Source: CAD feature listing. Evaluate the final solid. Frame: model axes, mm. Face numbers are marked on the shaded views. A direction names the side the tool comes from. Round coordinates to 2 decimals unless told otherwise and drop trailing zeros. Loops run counter-clockwise (first coordinate to the right, second up) from the corner with the lowest first, then second, coordinate; pieces in that order, holes last.
Item 1: Section query A-A on z = 13.75. Return loops of the section in (x, y).
Item 2: Section query C-C on y = 9.5. Return loops of the section in (x, z).
Item 3: Section query D-D on x = -9. Return loops of the section in (y, z).
Item 4: First-contact query: P1, Ø5, axis at x = 2, y = 0.5, coming from the +Z side; P2, Ø4, axis at x = 36, y = 3, coming from the +Z side; P3, Ø8, axis at x = -15.5, z = 3, coming from the -Y side; P4, Ø1.5, axis at y = 7, z = 14, coming from the -X side. Flat tips, straight axial feed; report the tip coordinate or a pass-through.
Item 5: Ray query, L1, parallel to Y at x = -43.5, z = 2.1; L2, parallel to Y at x = -3, z = 13; L3, parallel to X at y = 1, z = 6.75. Return the intervals inside material, ascending.
Item 6: Section query B-B on x = -43.5. Return loops of the section in (y, z), then the cut area to 3 significant figures.
Item 7: Access query for the marked faces 1, 2 and 3. Directions: +Z, -Z, +X, -X, +Y, -Y. A direction counts if a zero-diameter tool reaches every point of the face in a straight line with its end or side. Return the directions, or none.
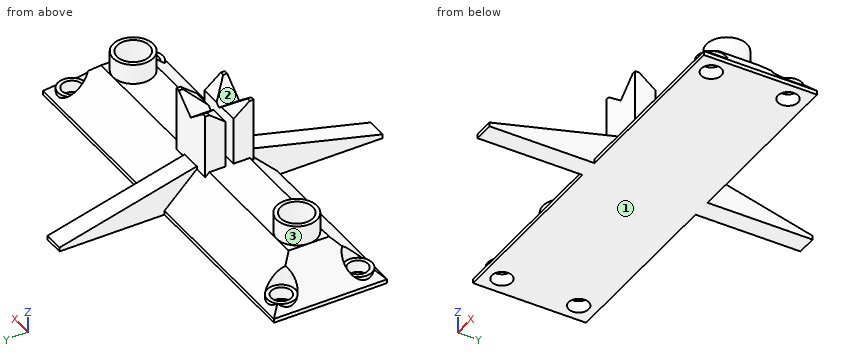
```python
from build123d import *

# Parameters (mm, degrees)
F0_R         = 3.5
F0_R_2       = 5
F0_W         = 5
F0_H         = 26
F0_W_2       = 2.5
F0_H_2       = 6
F0_W_3       = 3.5
F1_DEPTH     = 10
F0_R_3       = 4
F2_DEPTH     = 15
F3_DEPTH     = 1
F4_T4_DEPTH  = 74.2902937834
F4_S5_R      = 5
F4_T6_DEPTH  = 39
F4_T10_DEPTH = 74.2902937834
F4_S11_R     = 5
F4_T12_DEPTH = 39
F4_T16_DEPTH = 91.7902937834
F4_T21_DEPTH = 68.6451468917
F4_S22_R     = 5
F4_T23_DEPTH = 36
F4_T27_DEPTH = 68.6451468917
F4_S28_R     = 5
F4_T29_DEPTH = 36
F4_T33_DEPTH = 91.7902937834
F4_T38_DEPTH = 91.7902937834
F4_T43_DEPTH = 68.6451468917
F4_S44_R     = 5
F4_T45_DEPTH = 36
F4_T49_DEPTH = 68.6451468917
F4_S50_R     = 5
F4_T51_DEPTH = 36
F4_T55_DEPTH = 91.7902937834
F5_SIZE2     = 9
F5_SIZE      = 35
F0_R_4       = 2.5
F6_DEPTH     = 3
F7_DEPTH     = 25
F8_W         = 2
F8_H         = 7
F10_DEPTH    = 25
F11_DEPTH    = 25


# Not quite as in the source:
# - a fillet or chamfer that OpenCascade refuses, or shapes differently, is made with other operations: its cross-section is extruded or revolved along the edge and cut away or added


with BuildPart() as f1:
    # F0 (on Top) → F1 (new body)
    with BuildSketch(Plane.XY):
        Polygon((-2.5, 14), (-48, 14), (-48, -14), (-2.5, -14), (-2.5, -6), (-6, -6), (-6, 0), (-6, 6), (-2.5, 6), align=None)
        with Locations((-43.5, -9.5)):
            Circle(F0_R, mode=Mode.SUBTRACT)
        with Locations((-43.5, 9.5)):
            Circle(F0_R, mode=Mode.SUBTRACT)
        with Locations((-34, 0)):
            Circle(F0_R_2, mode=Mode.SUBTRACT)
        Polygon((48, 14), (2.5, 14), (2.5, 6), (6, 6), (6, 0), (6, -6), (2.5, -6), (2.5, -14), (48, -14), align=None)
        with Locations((43.5, -9.5)):
            Circle(F0_R, mode=Mode.SUBTRACT)
        with Locations((34, 0)):
            Circle(F0_R_2, mode=Mode.SUBTRACT)
        with Locations((43.5, 9.5)):
            Circle(F0_R, mode=Mode.SUBTRACT)
        Polygon((-2.5, -6), (-2.5, -14), (2.5, -14), (2.5, -6), (0, -6), align=None)
        with Locations((0, -27)):
            Rectangle(F0_W, F0_H)
        Polygon((2.5, 14), (-2.5, 14), (-2.5, 6), (0, 6), (2.5, 6), align=None)
        with Locations((0, 27)):
            Rectangle(F0_W, F0_H)
        with Locations((1.25, -3)):
            Rectangle(F0_W_2, F0_H_2)
        with Locations((4.25, -3)):
            Rectangle(F0_W_3, F0_H_2)
        with Locations((-4.25, -3)):
            Rectangle(F0_W_3, F0_H_2)
        with Locations((-1.25, -3)):
            Rectangle(F0_W_2, F0_H_2)
        with Locations((-1.25, 3)):
            Rectangle(F0_W_2, F0_H_2)
        with Locations((-4.25, 3)):
            Rectangle(F0_W_3, F0_H_2)
        with Locations((4.25, 3)):
            Rectangle(F0_W_3, F0_H_2)
        with Locations((1.25, 3)):
            Rectangle(F0_W_2, F0_H_2)
    extrude(amount=F1_DEPTH)

    # F0 (on Top) → F2 (join)
    with BuildSketch(Plane.XY):
        with Locations((-34, 0)):
            Circle(F0_R_2)
        with Locations((-34, 0)):
            Circle(F0_R_3, mode=Mode.SUBTRACT)
        with Locations((34, 0)):
            Circle(F0_R_2)
        with Locations((34, 0)):
            Circle(F0_R_3, mode=Mode.SUBTRACT)
    extrude(amount=F2_DEPTH)

    # F0 (on Top) → F3 (join)
    with BuildSketch(Plane.XY):
        with Locations((-34, 0)):
            Circle(F0_R_3)
        with Locations((34, 0)):
            Circle(F0_R_3)
    extrude(amount=F3_DEPTH)

    # F4: chamfer of 9 on 6 edges, made by hand


with BuildPart() as f4_tool2:
    # F4_s3 → F4_t4 (new body)
    with BuildSketch(Plane.XZ.offset(37.1451468917)):
        Polygon((39, 10), (48, 1), (48, 10), align=None)
    extrude(amount=-F4_T4_DEPTH)

    # F4_s5 → F4_t6 (cut, symmetric)
    with BuildSketch(Plane.XY.offset(5.5)):
        with Locations((34, 0)):
            Circle(F4_S5_R)
    extrude(amount=F4_T6_DEPTH, both=True, mode=Mode.SUBTRACT)


with BuildPart() as f1_1:
    add(f1.part)

    # F4_t1: cut F4_tool2
    add(f4_tool2.part, mode=Mode.SUBTRACT)


with BuildPart() as f4_tool8:
    # F4_s9 → F4_t10 (new body)
    with BuildSketch(Plane.XZ.offset(-37.1451468917)):
        Polygon((-48, 1), (-39, 10), (-48, 10), align=None)
    extrude(amount=F4_T10_DEPTH)

    # F4_s11 → F4_t12 (cut, symmetric)
    with BuildSketch(Plane.XY.offset(5.5)):
        with Locations((-34, 0)):
            Circle(F4_S11_R)
    extrude(amount=F4_T12_DEPTH, both=True, mode=Mode.SUBTRACT)


with BuildPart() as f1_2:
    add(f1_1.part)

    # F4_t7: cut F4_tool8
    add(f4_tool8.part, mode=Mode.SUBTRACT)


with BuildPart() as f4_tool14:
    # F4_s15 → F4_t16 (new body)
    with BuildSketch(Plane.YZ.offset(20.6451468917)):
        Polygon((14, 1), (5, 10), (14, 10), align=None)
    extrude(amount=-F4_T16_DEPTH)

    split(bisect_by=Plane.YZ.offset(2.5), keep=Keep.TOP)


with BuildPart() as f1_3:
    add(f1_2.part)

    # F4_t13: cut F4_tool14
    add(f4_tool14.part, mode=Mode.SUBTRACT)


with BuildPart() as f4_tool19:
    # F4_s20 → F4_t21 (new body)
    with BuildSketch(Plane.YZ.offset(-2.5)):
        Polygon((14, 1), (5, 10), (14, 10), align=None)
    extrude(amount=-F4_T21_DEPTH)

    # F4_s22 → F4_t23 (cut, symmetric)
    with BuildSketch(Plane.XY.offset(5.5)):
        with Locations((-34, 0)):
            Circle(F4_S22_R)
    extrude(amount=F4_T23_DEPTH, both=True, mode=Mode.SUBTRACT)


with BuildPart() as f1_4:
    add(f1_3.part)

    # F4_t18: cut F4_tool19
    add(f4_tool19.part, mode=Mode.SUBTRACT)


with BuildPart() as f4_tool25:
    # F4_s26 → F4_t27 (new body)
    with BuildSketch(Plane.YZ.offset(71.1451468917)):
        Polygon((5, 10), (14, 1), (14, 10), align=None)
    extrude(amount=-F4_T27_DEPTH)

    # F4_s28 → F4_t29 (cut, symmetric)
    with BuildSketch(Plane.XY.offset(5.5)):
        with Locations((34, 0)):
            Circle(F4_S28_R)
    extrude(amount=F4_T29_DEPTH, both=True, mode=Mode.SUBTRACT)


with BuildPart() as f1_5:
    add(f1_4.part)

    # F4_t24: cut F4_tool25
    add(f4_tool25.part, mode=Mode.SUBTRACT)


with BuildPart() as f4_tool31:
    # F4_s32 → F4_t33 (new body)
    with BuildSketch(Plane.YZ.offset(71.1451468917)):
        Polygon((5, 10), (14, 1), (14, 10), align=None)
    extrude(amount=-F4_T33_DEPTH)

    split(bisect_by=Plane.YZ.offset(-2.5), keep=Keep.BOTTOM)


with BuildPart() as f1_6:
    add(f1_5.part)

    # F4_t30: cut F4_tool31
    add(f4_tool31.part, mode=Mode.SUBTRACT)


with BuildPart() as f4_tool36:
    # F4_s37 → F4_t38 (new body)
    with BuildSketch(Plane.YZ.offset(-20.6451468917)):
        Polygon((-5, 10), (-14, 1), (-14, 10), align=None)
    extrude(amount=F4_T38_DEPTH)

    split(bisect_by=Plane.YZ.offset(-2.5), keep=Keep.BOTTOM)


with BuildPart() as f1_7:
    add(f1_6.part)

    # F4_t35: cut F4_tool36
    add(f4_tool36.part, mode=Mode.SUBTRACT)


with BuildPart() as f4_tool41:
    # F4_s42 → F4_t43 (new body)
    with BuildSketch(Plane.YZ.offset(2.5)):
        Polygon((-5, 10), (-14, 1), (-14, 10), align=None)
    extrude(amount=F4_T43_DEPTH)

    # F4_s44 → F4_t45 (cut, symmetric)
    with BuildSketch(Plane.XY.offset(5.5)):
        with Locations((34, 0)):
            Circle(F4_S44_R)
    extrude(amount=F4_T45_DEPTH, both=True, mode=Mode.SUBTRACT)


with BuildPart() as f1_8:
    add(f1_7.part)

    # F4_t40: cut F4_tool41
    add(f4_tool41.part, mode=Mode.SUBTRACT)


with BuildPart() as f4_tool47:
    # F4_s48 → F4_t49 (new body)
    with BuildSketch(Plane.YZ.offset(-71.1451468917)):
        Polygon((-14, 1), (-5, 10), (-14, 10), align=None)
    extrude(amount=F4_T49_DEPTH)

    # F4_s50 → F4_t51 (cut, symmetric)
    with BuildSketch(Plane.XY.offset(5.5)):
        with Locations((-34, 0)):
            Circle(F4_S50_R)
    extrude(amount=F4_T51_DEPTH, both=True, mode=Mode.SUBTRACT)


with BuildPart() as f1_9:
    add(f1_8.part)

    # F4_t46: cut F4_tool47
    add(f4_tool47.part, mode=Mode.SUBTRACT)


with BuildPart() as f4_tool53:
    # F4_s54 → F4_t55 (new body)
    with BuildSketch(Plane.YZ.offset(-71.1451468917)):
        Polygon((-14, 1), (-5, 10), (-14, 10), align=None)
    extrude(amount=F4_T55_DEPTH)

    split(bisect_by=Plane.YZ.offset(2.5), keep=Keep.TOP)


with BuildPart() as f1_10:
    add(f1_9.part)

    # F4_t52: cut F4_tool53
    add(f4_tool53.part, mode=Mode.SUBTRACT)

    # F5
    f5_edges = [f1_10.edges().sort_by_distance(p)[0] for p in [
        (0, 40, 10),
        (0, -40, 10),
    ]]
    f5_side = f1_10.faces().sort_by_distance((0, 0, 10))[0]
    chamfer(f5_edges, length=F5_SIZE, length2=F5_SIZE2, reference=f5_side)

    # F0 (on Top) → F6 (join)
    with BuildSketch(Plane.XY):
        with Locations((-43.5, -9.5)):
            Circle(F0_R)
        with Locations((-43.5, -9.5)):
            Circle(F0_R_4, mode=Mode.SUBTRACT)
        with Locations((-43.5, 9.5)):
            Circle(F0_R)
        with Locations((-43.5, 9.5)):
            Circle(F0_R_4, mode=Mode.SUBTRACT)
        with Locations((43.5, 9.5)):
            Circle(F0_R)
        with Locations((43.5, 9.5)):
            Circle(F0_R_4, mode=Mode.SUBTRACT)
        with Locations((43.5, -9.5)):
            Circle(F0_R)
        with Locations((43.5, -9.5)):
            Circle(F0_R_4, mode=Mode.SUBTRACT)
    extrude(amount=F6_DEPTH)

    # F0 (on Top) → F7 (join)
    with BuildSketch(Plane.XY):
        with Locations((4.25, -3)):
            Rectangle(F0_W_3, F0_H_2)
        with Locations((1.25, -3)):
            Rectangle(F0_W_2, F0_H_2)
        with Locations((-1.25, -3)):
            Rectangle(F0_W_2, F0_H_2)
        with Locations((-4.25, -3)):
            Rectangle(F0_W_3, F0_H_2)
        with Locations((-4.25, 3)):
            Rectangle(F0_W_3, F0_H_2)
        with Locations((-1.25, 3)):
            Rectangle(F0_W_2, F0_H_2)
        with Locations((4.25, 3)):
            Rectangle(F0_W_3, F0_H_2)
        with Locations((1.25, 3)):
            Rectangle(F0_W_2, F0_H_2)
    extrude(amount=F7_DEPTH)

    # F8 (on face) → F10 (cut)
    with BuildSketch(Plane.YZ.offset(6)):
        Polygon((-1, 25), (-5, 25), (-1, 21.8), align=None)
        Polygon((-1, 25), (-1, 21.8), (0, 21), (1, 21.8), (1, 25), align=None)
        Polygon((5, 25), (1, 25), (1, 21.8), align=None)
        Polygon((0, 21), (-1, 21.8), (-1, 17), (1, 17), (1, 21.8), align=None)
        with Locations((0, 13.5)):
            Rectangle(F8_W, F8_H)
    extrude(amount=-F10_DEPTH, mode=Mode.SUBTRACT)

    # F9 (on face) → F11 (cut)
    with BuildSketch(Plane.XZ.offset(6)):
        Polygon((-1, 25), (-1, 21.8), (0, 21), (1, 21.8), (1, 25), align=None)
        Polygon((-1, 25), (-5, 25), (-1, 21.8), align=None)
        Polygon((5, 25), (1, 25), (1, 21.8), align=None)
    extrude(amount=-F11_DEPTH, mode=Mode.SUBTRACT)


solid = f1_10.part
```
Data:
1. outline: circle Ø10 at (-34, 0); (-6, -6) - (6, -6) - (6, -1) - (-6, -1) - close; (-6, 1) - (6, 1) - (6, 6) - (-6, 6) - close; circle Ø10 at (34, 0); hole circle Ø8 at (-34, 0); hole circle Ø8 at (34, 0)
2. outline: (-48, 0) - (-46, 0) - (-46, 3) - (-47, 3) - (-47, 2) - (-48, 1) - close; (-41, 0) - (41, 0) - (41, 3) - (40, 3) - (40, 5.5) - (2.5, 5.5) - (2.5, 8.84) - (-2.5, 8.84) - (-2.5, 5.5) - (-40, 5.5) - (-40, 3) - (-41, 3) - close; (46, 0) - (48, 0) - (48, 1) - (47, 2) - (47, 3) - (46, 3) - close
3. outline: (-14, 0) - (14, 0) - (14, 1) - (5, 10) - (-5, 10) - (-14, 1) - close
4. P1: stops at z = 23.28
4. P2: stops at z = 15
4. P3: stops at y = -14
4. P4: passes through
5. L1: y = -13 to -12, -7 to 7, 12 to 13
5. L2: y = -6 to -1, 1 to 6
5. L3: x = -42.25 to -37.87, -30.13 to 30.13, 37.87 to 42.25
6. outline: (-14, 0) - (-12, 0) - (-12, 3) - (-13, 3) - (-13, 2) - (-14, 1) - close; (-7, 0) - (7, 0) - (7, 3) - (6, 3) - (6, 5.5) - (-6, 5.5) - (-6, 3) - (-7, 3) - close; (12, 0) - (14, 0) - (14, 1) - (13, 2) - (13, 3) - (12, 3) - close
6. area: 81.0 mm2
7. face 1: -Z, +X, -X, +Y, -Y
7. face 2: +Z, +Y, -Y
7. face 3: +Z
